Work out the finished part from the listing and answer in its coordinate system (mm). A direction names the side the tool comes from. Give positions to 0.01 mm unless a question says otherwise; leave off trailing zeros. Write each loop counter-clockwise with the first axis right and the second up, starting at its lowest first coordinate (ties: lowest second). Pieces come first, ordered by that corner, then holes. Notation, with made-up numbers: (5, 64.5) - (11, 64.5) arc R8 ccw to (11, 77.5) - close; hole circle Ø7 at (54, -15.75). An arc over 180 degrees is marked (long way). Write each question's results on one line, items separated by ' | '. Start each with the question number.
from build123d import *

# Parameters (mm, degrees)
F0_R            = 20
F1_DEPTH        = 10
F2_DEPTH        = 5
F3_DEPTH        = 5
F4_DEPTH        = 5
F5_DEPTH        = 5
F6_DEPTH        = 10
F7_DEPTH        = 10
F8_DEPTH        = 10
F9_DEPTH        = 10
F12_D           = 1
F12_DEPTH       = 20.001
F13_D           = 1
F13_DEPTH       = 20.0010001
F14_D           = 1
F15_D           = 1
F16_D           = 1
F16_CBORE_D     = 1.5
F16_CBORE_DEPTH = 1
F17_D           = 1
F17_CBORE_D     = 1.5
F17_CBORE_DEPTH = 1
F18_D           = 1
F18_CBORE_D     = 1.5
F18_CBORE_DEPTH = 1
F19_D           = 1
F19_CBORE_D     = 1.5
F19_CBORE_DEPTH = 1


with BuildPart() as f1:
    # F0 (on Top) → F1 (new body)
    with BuildSketch(Plane.XY):
        Circle(F0_R)
        with BuildLine():
            ThreePointArc((-16.237976321, -9.375), (-18.75, 0), (-16.237976321, 9.375))
            ThreePointArc((-16.237976321, 9.375), (-13.2582521472, 13.2582521472), (-9.375, 16.237976321))
            ThreePointArc((-9.375, 16.237976321), (0, 18.75), (9.375, 16.237976321))
            ThreePointArc((9.375, 16.237976321), (13.2582521472, 13.2582521472), (16.237976321, 9.375))
            ThreePointArc((16.237976321, 9.375), (18.75, 0), (16.237976321, -9.375))
            ThreePointArc((16.237976321, -9.375), (13.2582521472, -13.2582521472), (9.375, -16.237976321))
            ThreePointArc((9.375, -16.237976321), (0, -18.75), (-9.375, -16.237976321))
            ThreePointArc((-9.375, -16.237976321), (-13.2582521472, -13.2582521472), (-16.237976321, -9.375))
        make_face(mode=Mode.SUBTRACT)
    extrude(amount=F1_DEPTH)

    # F0 (on Top) → F2 (join)
    with BuildSketch(Plane.XY):
        with BuildLine():
            ThreePointArc((-15.1554445662, -8.75), (-17.5, 0), (-15.1554445662, 8.75))
            Line((-15.1554445662, 8.75), (-16.237976321, 9.375))
            ThreePointArc((-16.237976321, 9.375), (-18.75, 0), (-16.237976321, -9.375))
            Line((-16.237976321, -9.375), (-15.1554445662, -8.75))
        make_face()
    extrude(amount=F2_DEPTH)

    # F0 (on Top) → F3 (join)
    with BuildSketch(Plane.XY):
        with BuildLine():
            Line((-9.375, 16.237976321), (-8.75, 15.1554445662))
            ThreePointArc((-8.75, 15.1554445662), (0, 17.5), (8.75, 15.1554445662))
            Line((8.75, 15.1554445662), (9.375, 16.237976321))
            ThreePointArc((9.375, 16.237976321), (0, 18.75), (-9.375, 16.237976321))
        make_face()
    extrude(amount=F3_DEPTH)

    # F0 (on Top) → F4 (join)
    with BuildSketch(Plane.XY):
        with BuildLine():
            ThreePointArc((8.75, -15.1554445662), (0, -17.5), (-8.75, -15.1554445662))
            Line((-8.75, -15.1554445662), (-9.375, -16.237976321))
            ThreePointArc((-9.375, -16.237976321), (0, -18.75), (9.375, -16.237976321))
            Line((9.375, -16.237976321), (8.75, -15.1554445662))
        make_face()
    extrude(amount=F4_DEPTH)

    # F0 (on Top) → F5 (join)
    with BuildSketch(Plane.XY):
        with BuildLine():
            Line((16.237976321, 9.375), (15.1554445662, 8.75))
            ThreePointArc((15.1554445662, 8.75), (17.5, 0), (15.1554445662, -8.75))
            Line((15.1554445662, -8.75), (16.237976321, -9.375))
            ThreePointArc((16.237976321, -9.375), (18.75, 0), (16.237976321, 9.375))
        make_face()
    extrude(amount=F5_DEPTH)

    # F0 (on Top) → F6 (join)
    with BuildSketch(Plane.XY):
        with BuildLine():
            Line((-16.237976321, 9.375), (-15.1554445662, 8.75))
            ThreePointArc((-15.1554445662, 8.75), (-12.3743686708, 12.3743686708), (-8.75, 15.1554445662))
            Line((-8.75, 15.1554445662), (-9.375, 16.237976321))
            ThreePointArc((-9.375, 16.237976321), (-13.2582521472, 13.2582521472), (-16.237976321, 9.375))
        make_face()
    extrude(amount=F6_DEPTH)

    # F0 (on Top) → F7 (join)
    with BuildSketch(Plane.XY):
        with BuildLine():
            ThreePointArc((-8.75, -15.1554445662), (-12.3743686708, -12.3743686708), (-15.1554445662, -8.75))
            Line((-15.1554445662, -8.75), (-16.237976321, -9.375))
            ThreePointArc((-16.237976321, -9.375), (-13.2582521472, -13.2582521472), (-9.375, -16.237976321))
            Line((-9.375, -16.237976321), (-8.75, -15.1554445662))
        make_face()
    extrude(amount=F7_DEPTH)

    # F0 (on Top) → F8 (join)
    with BuildSketch(Plane.XY):
        with BuildLine():
            ThreePointArc((15.1554445662, -8.75), (12.3743686708, -12.3743686708), (8.75, -15.1554445662))
            Line((8.75, -15.1554445662), (9.375, -16.237976321))
            ThreePointArc((9.375, -16.237976321), (13.2582521472, -13.2582521472), (16.237976321, -9.375))
            Line((16.237976321, -9.375), (15.1554445662, -8.75))
        make_face()
    extrude(amount=F8_DEPTH)

    # F0 (on Top) → F9 (join)
    with BuildSketch(Plane.XY):
        with BuildLine():
            Line((9.375, 16.237976321), (8.75, 15.1554445662))
            ThreePointArc((8.75, 15.1554445662), (12.3743686708, 12.3743686708), (15.1554445662, 8.75))
            Line((15.1554445662, 8.75), (16.237976321, 9.375))
            ThreePointArc((16.237976321, 9.375), (13.2582521472, 13.2582521472), (9.375, 16.237976321))
        make_face()
    extrude(amount=F9_DEPTH)

    # F12 (through all, one way)
    with BuildSketch(Plane.YZ):
        with Locations((0, 7.4741876426)):
            Circle(F12_D / 2)
    extrude(amount=-F12_DEPTH, mode=Mode.SUBTRACT)

    # F13 (through all, one way)
    with BuildSketch(Plane.XZ):
        with Locations((0, 7.5)):
            Circle(F13_D / 2)
    extrude(amount=-F13_DEPTH, mode=Mode.SUBTRACT)

    # F14 (through all)
    with Locations(Plane(origin=(0, 0, 0), x_dir=(1, 0, 0), z_dir=(0, 1, 0))):
        with Locations((0, -7.5)):
            Hole(F14_D / 2)

    # F15 (through all)
    with Locations(Plane(origin=(0, 0, 0), x_dir=(0, 1, 0), z_dir=(-1, 0, 0))):
        with Locations((0, -7.4741876426)):
            Hole(F15_D / 2)

    # F16 (through all)
    with Locations(Plane(origin=(0, 0, 0), x_dir=(1, 0, 0), z_dir=(0, 0, -1))):
        with Locations((-13.2582521472, 13.2582521472)):
            CounterBoreHole(F16_D / 2, F16_CBORE_D / 2, F16_CBORE_DEPTH)

    # F17 (through all)
    with Locations(Plane(origin=(0, 0, 0), x_dir=(1, 0, 0), z_dir=(0, 0, -1))):
        with Locations((13.2582521472, 13.2582521472)):
            CounterBoreHole(F17_D / 2, F17_CBORE_D / 2, F17_CBORE_DEPTH)

    # F18 (through all)
    with Locations(Plane(origin=(0, 0, 0), x_dir=(1, 0, 0), z_dir=(0, 0, -1))):
        with Locations((13.2582521472, -13.2582521472)):
            CounterBoreHole(F18_D / 2, F18_CBORE_D / 2, F18_CBORE_DEPTH)

    # F19 (through all)
    with Locations(Plane(origin=(0, 0, 0), x_dir=(1, 0, 0), z_dir=(0, 0, -1))):
        with Locations((-13.2582521472, -13.2582521472)):
            CounterBoreHole(F19_D / 2, F19_CBORE_D / 2, F19_CBORE_DEPTH)


solid = f1.part
Q1. A cutting plane is placed at A-A, the plane y = 0. Write down the section's boundary in (x, z), and give its area (3 significant figures).
Q2. Given pin 1 (1.7 mm diameter, centred on x = 13.26, y = -13.26, fed in from -Z); pin 2 (1.8 mm diameter, centred on x = -16, y = 1, fed in from +Z); pin 3 (4 mm diameter, centred on x = 14.5, z = 7.5, fed in from -Y); pin 4 (1.8 mm diameter, centred on x = 17.5, y = 1, fed in from +Z), each flat-ended and moving along its own axis, determine where each tip first touches the part or whether it passes through.
Q3. A cutting plane is placed at D-D, the plane y = 11.5. Write down the section's boundary in (x, z).
Q4. Consider L1, parallel to Y at x = 13, z = 6.5; L2, parallel to Z at x = 19.4, y = 0; L3, parallel to X at y = -13.5, z = 6.75. Determine where each line is inside the solid, lowest interval first.
Q5. A cutting plane is placed at C-C, the plane z = 3. Write down the section's boundary in (x, y), and give its area (3 significant figures).
Q6. The mould has two halves that part along X. Classify faces 4 (the flat face through (0, -18, 0)), 5 (the flat face through (-9.067, -15.704, 7.465)), 6 (the cylindrical face through (-4.336, -19.524, 4.93)): pulls with the +X half, pulls with the -X half, needs draft (parallel to the pull), parting line crosses it, or undercut.
Q7. A tool of negligible diameter and unlimited length cuts with its end or side. For faces 1 (the cylindrical face through (-13.489, -12.815, 5.563)), 2 (the flat face through (-9.06, 15.69, 7.46)), 3 (the cylindrical face through (12.51, -13.29, 0.49)), from which of +Z, -Z, +X, -X, +Y, -Y can it reach the whole face along a straight path? Write none if from no direction.
Q8. A cutting plane is placed at B-B, the plane x = -1. Write down the section's boundary in (y, z).
Result:
1) outline: (-20, 0) - (-17.5, 0) - (-17.5, 5) - (-18.75, 5) - (-18.75, 6.97) - (-20, 6.97) - close; (-20, 7.97) - (-18.75, 7.97) - (-18.75, 10) - (-20, 10) - close; (17.5, 0) - (20, 0) - (20, 6.97) - (18.75, 6.97) - (18.75, 5) - (17.5, 5) - close; (18.75, 7.97) - (20, 7.97) - (20, 10) - (18.75, 10) - close | area: 35.0 mm2
2) pin 1: stops at z = 0 | pin 2: passes through | pin 3: stops at y = -15.61 | pin 4: stops at z = 5
3) outline: (-16.36, 0) - (-13.19, 0) - (-13.19, 10) - (-16.36, 10) - close; (13.19, 0) - (16.36, 0) - (16.36, 10) - (13.19, 10) - close
4) L1: y = -15.2 to -13.69, -12.83 to -11.72, 11.72 to 12.83, 13.69 to 15.2 | L2: z = 0 to 6.97, 7.97 to 10 | L3: x = -14.76 to -13.7, -12.82 to -11.14, 11.14 to 12.82, 13.7 to 14.76
5) outline: circle Ø40 at (0, 0); hole circle Ø35 at (0, 0); hole circle Ø1 at (-13.26, -13.26); hole circle Ø1 at (-13.26, 13.26); hole circle Ø1 at (13.26, -13.26); hole circle Ø1 at (13.26, 13.26) | area: 291 mm2
6) face 4: needs draft | face 5: undercut | face 6: parting line crosses it
7) face 1: +Z, -Z | face 2: +Z | face 3: -Z
8) outline: (-19.97, 0) - (-17.47, 0) - (-17.47, 5) - (-18.72, 5) - (-18.72, 10) - (-19.97, 10) - close; (17.47, 0) - (19.97, 0) - (19.97, 10) - (18.72, 10) - (18.72, 5) - (17.47, 5) - close
